from build123d import *

# Parameters (mm, degrees)
F2_R     = 1.5875
F3_DEPTH = 152.4
F5_DEPTH = 5.08


with BuildPart() as f1:
    # F0 (on Front) → F1 (revolve)
    with BuildSketch(Plane.XZ):
        with BuildLine():
            Line((0, 76.2), (0, 0))
            ThreePointArc((0, 0), (7.4556115815, 0.963776837), (12.7, 6.35))
            Line((12.7, 6.35), (12.7, 76.2))
            Line((12.7, 76.2), (0, 76.2))
        make_face()
    revolve(axis=Axis((0, 0, 38.1), (0, 0, 1)))

    # F2 (on Top) → F3 (join)
    with BuildSketch(Plane.XY):
        Circle(F2_R)
    extrude(amount=F3_DEPTH)

    # F4 (on face) → F5 (join)
    with BuildSketch(Plane.XY.offset(152.4)):
        with BuildLine():
            Line((1.5242467692, 0.4436530587), (-1.5242467692, 0.4436530587))
            ThreePointArc((-1.5242467692, 0.4436530587), (-1.5873331828, -0.0230134024), (-1.5107445232, -0.4876548326))
            Line((-1.5107445232, -0.4876548326), (1.5107445232, -0.4876548326))
            ThreePointArc((1.5107445232, -0.4876548326), (1.5681937349, -0.2468292117), (1.5875, 0))
            ThreePointArc((1.5875, 0), (1.5716071386, 0.2240697479), (1.5242467692, 0.4436530587))
        make_face()
    extrude(amount=F5_DEPTH)


solid = f1.part
The listing builds one solid part. Answer for the finished solid, in the listing's coordinates (mm). A direction names the side the tool comes from. Round coordinates to 2 decimals unless told otherwise and drop trailing zeros. Write each loop counter-clockwise with the first axis right and the second up, starting at its lowest first coordinate (ties: lowest second). Pieces come first, ordered by that corner, then holes. Notation, with made-up numbers: (79, -30.5) - (137, -30.5) arc R18 ccw to (137, -16.5) - close; hole circle Ø9 at (34, 36). An arc over 180 degrees is marked (long way). Use one line per item in the form item = value. Start each with the question number.
Item 1: A tool of negligible diameter and unlimited length cuts with its end or side. For faces 1 (the cylindrical face through (-2.75, -12.4, 41.76)), 2 (the flat face through (0, 0.444, 155)), 3 (the flat face through (0, -0.488, 155)), from which of +Z, -Z, +X, -X, +Y, -Y can it reach the whole face along a straight path? Write none if from no direction.
Item 2: A cutting plane is placed at B-B (z = 108). Write down the section's boundary in (x, y) (1 decimal).
Item 3: A cutting plane is placed at A-A (z = 27.5). Write down the section's boundary in (x, y), plus the area to 3 significant figures.
Item 4: Flat-ended cylindrical pins translate along their axes: pin 1 Ø1 at (y, z) = (1.5, 103.5) entering from +X; pin 2 Ø2.5 at (x, z) = (-0.5, 156) entering from +Y; pin 3 Ø2 at (y, z) = (-1.5, 17.5) entering from -X; pin 4 Ø12.5 at (x, y) = (-4, 2) entering from +Z. Find the tip coordinate at first contact, or state that the pin passes through.
Item 5: Find the intervals of material crossed by line 1 (Y direction, x = 0.5, z = 110); line 2 (Z direction, x = -5.75, y = 2.5); line 3 (X direction, y = -0.25, z = 11.5), in increasing order. Write a range as [from, to].
The answers:
q1.face_1 = +Z, -Z
q1.face_2 = +Z, +X, -X, +Y
q1.face_3 = +Z, +X, -X, -Y
q2.outline = circle Ø3.2 at (0, 0)
q3.outline = circle Ø25.4 at (0, 0)
q3.area = 507 mm^2
q4.pin_1 = 1.23
q4.pin_2 = 0.44
q4.pin_3 = -12.69
q4.pin_4 = 157.48
q5.line_1 = [-1.51, 1.51]
q5.line_2 = [0.45, 76.2]
q5.line_3 = [-12.7, 12.7]
